from build123d import *

# Parameters (mm, degrees)
RESSALTO_EXTRUS_O1_DEPTH = 50
ESBO_O2_R                = 1.5
CORTE_EXTRUS_O1_DEPTH    = 50


with BuildPart() as part:
    # Esboço1 → Ressalto-extrusão1 (new body)
    with BuildSketch(Plane.XY):
        Polygon((0, 0), (0, 27), (1.3, 27), (1.3, 7.5), (36, 7.5), (36, 6), (1.3, 6), (1.3, 1.3), (36, 1.3), (36, 0), align=None)
    extrude(amount=RESSALTO_EXTRUS_O1_DEPTH)

    # Esboço2 → Corte-extrusão1 (cut)
    with BuildSketch(Plane.ZY):
        with Locations((8.5, 14.5)):
            Circle(ESBO_O2_R)
        with Locations((41.5, 14.5)):
            Circle(ESBO_O2_R)
        with BuildLine():
            Line((0, 20), (3.35, 20))
            ThreePointArc((3.35, 20), (5, 18.35), (3.35, 16.7))
            Line((3.35, 16.7), (0, 16.7))
            Line((0, 16.7), (0, 20))
        make_face()
        with BuildLine():
            Line((50, 16.7), (50, 20))
            Line((50, 20), (46.65, 20))
            ThreePointArc((46.65, 20), (45, 18.35), (46.65, 16.7))
            Line((46.65, 16.7), (50, 16.7))
        make_face()
    extrude(amount=-CORTE_EXTRUS_O1_DEPTH, mode=Mode.SUBTRACT)


solid = part.part
Could you check a few things on this model? Use its own coordinates, in mm. A direction names the side the tool comes from. Coordinates: 2 decimals unless noted, no trailing zeros. Write each loop counter-clockwise with the first axis right and the second up, starting at its lowest first coordinate (ties: lowest second). Pieces come first, ordered by that corner, then holes. Notation, with made-up numbers: (71.5, 30.25) - (117.5, 30.25) arc R19 cw to (117.5, 62.25) - close; hole circle Ø10 at (19.5, 25.5). An arc over 180 degrees is marked (long way). Write item = value, one per line.
1) Please list where these lines run through material, in increasing order: line 1 (Y direction, x = 0.5, z = 8.5); line 2 (Y direction, x = 14, z = 14); line 3 (X direction, y = 12.75, z = 33.5). Write a range as [from, to].
Result set:
line_1 = [0, 13], [16, 27]
line_2 = [0, 1.3], [6, 7.5]
line_3 = [0, 1.3]
2) Suppose I cut it at D-D on z = 14.5. Please give me the cut outline in (x, y), plus the area to 3 significant figures.
Result set:
outline = (0, 0) - (36, 0) - (36, 1.3) - (1.3, 1.3) - (1.3, 6) - (36, 6) - (36, 7.5) - (1.3, 7.5) - (1.3, 27) - (0, 27) - close
area = 132 mm2
3) For faces 5 (the flat face through (1, 20, 2)), 6 (the flat face through (1.3, 4, 25)), 7 (the flat face through (18, 7.5, 25)), which set-ups out of +Z, -Z, +X, -X, +Y, -Y let a thin tool reach every point of the face, with its end or its side?
Result set:
face_5 = -Z, +X, -X
face_6 = +Z, -Z, +X
face_7 = +Z, -Z, +X, +Y
4) Suppose I cut it at C-C on x = 21.5. Please give me the cut outline in (y, z), plus the area to 3 significant figures.
Result set:
outline = (0, 0) - (1.3, 0) - (1.3, 50) - (0, 50) - close; (6, 0) - (7.5, 0) - (7.5, 50) - (6, 50) - close
area = 140 mm2
5) Suppose I cut it at A-A on z = 8.5. Please give me the cut outline in (x, y), plus the area to 3 significant figures.
Result set:
outline = (0, 0) - (36, 0) - (36, 1.3) - (1.3, 1.3) - (1.3, 6) - (36, 6) - (36, 7.5) - (1.3, 7.5) - (1.3, 13) - (0, 13) - close; (0, 16) - (1.3, 16) - (1.3, 27) - (0, 27) - close
area = 128 mm2
6) Suppose I cut it at B-B on y = 14.5. Please give me the cut outline in (x, z).
Result set:
outline = (0, 0) - (1.3, 0) - (1.3, 7) - (0, 7) - close; (0, 10) - (1.3, 10) - (1.3, 40) - (0, 40) - close; (0, 43) - (1.3, 43) - (1.3, 50) - (0, 50) - close
7) Will these pins go through, and if not, where does the flat tip stop? pin 1 Ø1.8 at (y, z) = (14.5, 41.5) entering from +X; pin 2 Ø1 at (y, z) = (24, 40) entering from +X; pin 3 Ø10.5 at (x, z) = (10, 15.5) entering from +Y; pin 4 Ø1 at (x, z) = (0.5, 48) entering from -Y.
Result set:
pin_1 = through
pin_2 = 1.3
pin_3 = 7.5
pin_4 = 0
8) We'd pull the mould along Z, two halves only. Please class faces 1 (the cylindrical face through (0.6, 18.4, 45)), 2 (the flat face through (18, 1.3, 25)), 3 (the flat face through (15, 7, 0)), 4 (the cylindrical face through (0.6, 13.6, 7.3)): +Z half, -Z half, draft (parallel to the pull), parting line (faces both ways), or undercut.
Result set:
face_1 = +Z half
face_2 = draft
face_3 = -Z half
face_4 = undercut
